from build123d import *

# Parameters (mm, degrees)
BOSS_EXTRUDE1_DEPTH = 6.8
FILLET1_R           = 12.7


with BuildPart() as part:
    # Sketch1 → Boss-Extrude1 (new body)
    with BuildSketch(Plane(origin=(0, 0, 0), x_dir=(1, 0, 0), z_dir=(0, 1, 0))):
        with BuildLine():
            Line((0, 0), (250, 0))
            Line((250, 0), (250, 50.8))
            ThreePointArc((250, 50.8), (125, 152.4), (0, 50.8))
            Line((0, 50.8), (0, 0))
        make_face()
    extrude(amount=BOSS_EXTRUDE1_DEPTH)

    # Fillet1
    fillet1_edges = [part.edges().sort_by_distance(p)[0] for p in [
        (0, 3.4, -50.8),
        (250, 3.4, -50.8),
    ]]
    fillet(fillet1_edges, radius=FILLET1_R)


solid = part.part
Build history of the part. All positions in model axes, mm. Coordinates: 2 decimals unless noted, no trailing zeros. Order: outer loops, then holes, each group sorted by start corner. A loop starts at its lowest first (then second) coordinate and runs counter-clockwise, first axis right, second up. Notation, with made-up numbers: M 76.5,6.5 L 122.5,6.5 A32 ccw 122.5,45.5 Z; hole C -25.5,-35.75 d2. An arc over 180 degrees is marked long. One line per question, with ' | ' between items. Start each with the question number.
Q1. Saw through at C-C (x = 85.5). List the corners of the cut face in (y, z).
Q2. Flat gauge pins, fed straight in: pin 1 Ø3 at (y, z) = (3, -67) entering from -X; pin 2 Ø3 at (y, z) = (1, -62) entering from -X. Where does each tip first touch, or does it go through?
Q3. Saw through at B-B (z = -99). List the corners of the cut face in (x, y).
Q4. Probe L1, parallel to X at y = 2.5, z = -83.5; L2, parallel to Z at x = 80, y = 4; L3, parallel to Z at x = 104, y = 4.5. List the from-to ranges inside material, lowest first. Write a range as from..to.
Q5. Saw through at A-A (y = 4). List the corners of the cut face in (x, z), then the cut area to 3 significant figures.
Check values:
1) outline: M 0,-146.14 L 6.8,-146.14 L 6.8,0 L 0,0 Z
2) pin 1: stops at x = 4 | pin 2: stops at x = 2.42
3) outline: M 21.14,0 L 228.86,0 L 228.86,6.8 L 21.14,6.8 Z
4) L1: x = 11.65..238.35 | L2: z = -144.21..0 | L3: z = -150.66..0
5) outline: M 0,-49.45 A12.7 ccw 0.3,-52.19 A127.69 ccw 249.7,-52.19 A12.7 ccw 250,-49.45 L 250,0 L 0,0 Z | area: 31,700 mm2
